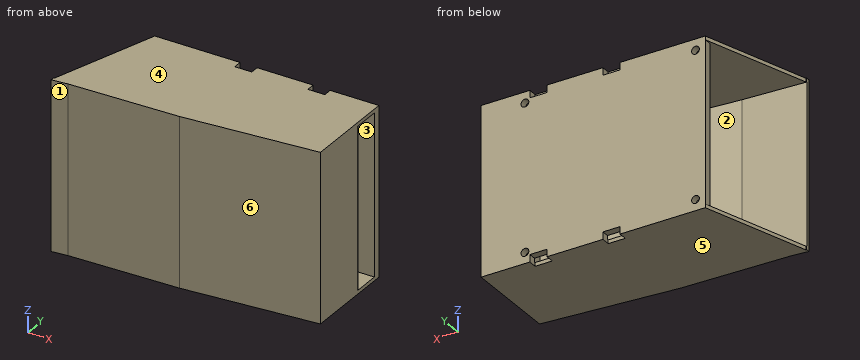
Autodesk Inventor part; units mm, degrees
ref_plane "工作平面1" through (0, 38.6, 0) normal (0, 1, 0) x (-1, 0, 0)
ref_plane "工作平面2" through (0, 0, 34.5) normal (0, 0, -1) x (-1, 0, 0)
ref_plane "工作平面3" through (0, -6, 0) normal (0, 1, 0) x (-1, 0, 0)
sketch "草图1" plane through (0, 0, 0) normal (0, 0, 1) x (1, 0, 0)
  line L0 (0, 0) -> (0, 3)
  line L1 (0, 0) -> (0, -6) construction
  line L2 (0, -6) -> (-106.5, -6) construction
  line L3 (-106.5, -6) -> (0, 3)
  line L4 (0, 0) -> (-54.9206, -4.6412)
  line L5 (-54.9206, -4.6412) -> (-106.5, -6)
  dimension "d0" = 3
  dimension "d1" = 6
  dimension "d2" = 106.5
extrude "拉伸1" add sketch "草图1" along normal blind 69
ref_plane "工作平面1" through (0, 38.6, 0) normal (0, 1, 0) x (-1, 0, 0)
sketch "草图2" plane through (0, 38.6, 0) normal (0, 1, 0) x (-1, 0, 0)
  line L0 (0, 0) -> (106.5, 0) construction
  line L1 (106.5, 0) -> (106.5, 69) construction
  line L2 (0, 69) -> (106.5, 69) construction
  line L3 (0, 0) -> (0, 69) construction
  line L4 (0, 0) -> (92, 0)
  line L5 (92, 0) -> (92, 1.5)
  line L6 (92, 1.5) -> (2, 1.5)
  line L7 (2, 1.5) -> (2, 67.5)
  line L8 (2, 67.5) -> (92, 67.5)
  line L9 (92, 67.5) -> (92, 69)
  line L10 (0, 0) -> (0, 69)
  line L11 (0, 69) -> (92, 69)
  line L12 (0, 69) -> (106.5, 69)
  line L13 (0, 0) -> (0, 69)
  dimension "d6" = 1.5
  dimension "d7" = 1.5
  dimension "d8" = 66
  dimension "d9" = 2
  dimension "d10" = 90
extrude "拉伸2" add sketch "草图2" against normal up to surface from surface at 0 surface through (0, 3, 0) normal (-0.0842069, 0.9964483, 0)
sketch "草图3" plane through (0, 38.6, 0) normal (0, 1, 0) x (-1, 0, 0)
  line L0 (2, 1.5) -> (92, 1.5) construction
  line L1 (2, 67.5) -> (2, 1.5) construction
  line L2 (92, 67.5) -> (2, 67.5) construction
  line L3 (92, 1.5) -> (2, 1.5)
  line L4 (2, 1.5) -> (2, 67.5)
  line L5 (92, 67.5) -> (2, 67.5)
  line L6 (92, 67.5) -> (92, 1.5)
  point P0 (0, 0)
extrude "拉伸3" add sketch "草图3" against normal blind 3
sketch "草图4" plane through (-2, 2.831, 1.5) normal (-1, 0, 0) x (0, 0, 1)
  line L0 (66, 32.769) -> (0, 32.769) construction
  line L1 (0, 0) -> (0, 32.769) construction
  line L2 (66, 0) -> (0, 0) construction
  line L3 (66, 0) -> (66, 32.769) construction
  line L4 (66, -7.6056) -> (66, 32.769)
  line L5 (0, 32.769) -> (66, 32.769)
  line L6 (66, 32.769) -> (66, 22.769)
  line L7 (66, 22.769) -> (0, 22.769)
  line L8 (0, 22.769) -> (0, 32.769)
  point P0 (-1.5, -2.831)
  dimension "d15" = 10
extrude "拉伸4" cut sketch "草图4" against normal through all
sketch "草图5" plane through (0, 0, 69) normal (0, 0, 1) x (1, 0, 0)
  line L0 (-92, -4.7746) -> (-92, 38.6) construction
  line L1 (-92, -4.7746) -> (-106.5, -6) construction
  line L2 (-92, 38.6) -> (-92, -4.7746)
  line L3 (-106.5, -6) -> (-54.9206, -4.6412)
  line L4 (-92, -4.7746) -> (-92, 35.6)
  line L5 (-106.5, -6) -> (-92, -4.7746)
  line L6 (-92, -4.7746) -> (-92, 38.6)
  line L7 (-106.5, -6) -> (-92, 38.6)
  point P0 (0, 0)
extrude "拉伸5" add sketch "草图5" against normal blind 1.5
ref_plane "工作平面2" through (0, 0, 34.5) normal (0, 0, -1) x (-1, 0, 0)
mirror "镜像1" about plane through (0, 0, 34.5) normal (0, 0, -1) of "拉伸5"
sketch "草图7" plane through (0, 38.6, 69) normal (0, 1, 0) x (1, 0, 0)
  line L0 (-92, 69) -> (0, 69)
  line L1 (0, 69) -> (0, 0) construction
  line L2 (0, 34.5) -> (-92.7255, 34.5) construction
  line L3 (-92, 1.5) -> (-92, 67.5)
  point P0 (-18, 64.5)
  point P1 (-52, 64.5)
  point P2 (-88, 64.5)
  point P3 (-18, 4.5)
  point P4 (-52, 4.5)
  point P5 (-88, 4.5)
  point P6 (-92, 66.5)
  dimension "d22" = 4.5
  dimension "d23" = 4.5
  dimension "d24" = 4.5
  dimension "d25" = 34
  dimension "d26" = 36
  dimension "d27" = 60
  dimension "d35" = 4
hole "孔1" at (-88, 38.6, 64.5) at (-88, 38.6, 4.5) at (-18, 38.6, 4.5) at (-18, 38.6, 64.5) direction (0, -1, 0) diameter 3.2 depth 3
fillet "圆角1" radius 1 1 edges at (0, 25.6, 34.5)
sketch "草图9" plane through (0, 0, 69) normal (0, 0, 1) x (1, 0, 0)
  point P0 (0, 0)
sketch "草图10" plane through (0, 0, 69) normal (0, 0, 1) x (1, 0, 0)
  line L0 (-92, 38.6) -> (-106.5, -6) construction
  line L1 (-92, 35.6) -> (-92, 38.6) construction
  line L2 (-92, -4.7746) -> (-92, 35.6) construction
  line L3 (-92, -4.7746) -> (-106.5, -6) construction
  line L4 (-106.5, -6) -> (-54.9206, -4.6412)
  line L5 (-106.5, -6) -> (-106.5, -5)
  line L6 (-127.8168, 0) -> (21.4009, 0)
  line L7 (-106.5, -5) -> (-80.7103, -3.8206)
  line L8 (-2, 2.831) -> (-106.5, -6)
  line L9 (-106.5, -6) -> (-92, 38.6)
  line L10 (-106.5, -6) -> (-80.7103, -3.8206)
  line L11 (-106.5, -6) -> (-106.5, -6.5)
  line L12 (-106.5, -6.5) -> (-80.7103, -3.8206)
  line L13 (-106.5, -5.2) -> (-80.7103, -3.8206)
  point P0 (0, 0)
  dimension "d37" = 1
  dimension "d38" = 25.7897
  dimension "d42" = 0.5
  dimension "d55" = 0.2
extrude "拉伸7" add sketch "草图10" against normal up to surface (69 mm away) from surface at 0 contours L8 L12 L4 | L9 L13 L8 | L5 L13 L9 | L4 L12 L11 | L5 L7 L9 L13 | L13 L9 L7
sketch "草图11" plane through (-54.9206, -4.6412, 0) normal (0.0263351, -0.9996532, 0) x (0.9996532, 0.0263351, 0)
  point P0 (55.0238, 0)
ref_plane "工作平面3" through (0, -6, 0) normal (0, 1, 0) x (-1, 0, 0)
sketch "草图12" plane through (0, 38.6, 69) normal (0, 1, 0) x (1, 0, 0)
  line L0 (0, 0) -> (-92, 0)
  line L1 (-53.5, 0) -> (-53.5, 3)
  line L2 (-92, 1.5) -> (-92, 67.5)
  line L3 (-54.9206, 0) -> (0, 0)
  line L4 (-57, 3) -> (-50, 3)
  line L5 (-50, 3) -> (-50, 0)
  line L6 (-50, 0) -> (-57, 0)
  line L7 (-57, 0) -> (-57, 3)
  line L8 (-92, 1.5) -> (0, 1.5)
  line L9 (-57, 3) -> (-50, 0) construction
  line L10 (-50, 3) -> (-57, 0) construction
  line L11 (-20, 3) -> (-27, 3)
  line L12 (-27, 3) -> (-27, 0)
  line L13 (-27, 0) -> (-20, 0)
  line L14 (-20, 0) -> (-20, 3)
  line L15 (-20, 3) -> (-27, 0) construction
  line L16 (-27, 3) -> (-20, 0) construction
  point P0 (0, 69)
  point P1 (-53.5, 1.5)
  point P2 (-23.5, 1.5)
  dimension "d43" = 38.5
  dimension "d44" = 3
  dimension "d45" = 7
  dimension "d46" = 68.5
  dimension "d47" = 3
  dimension "d48" = 7
extrude "拉伸8" cut sketch "草图12" against normal blind 3.5 contours L0 L12 L8 L14 | L8 L12 L11 L14 | L0 L1 L8 L5 | L0 L7 L8 L1 | L8 L1 L4 L5 | L8 L7 L4 L1
ref_plane "工作平面4" through (0, 0, 34.5) normal (0, 0, 1) x (1, 0, 0)
mirror "镜像2" about plane through (0, 0, 34.5) normal (0, 0, 1) of "拉伸8"
extrude "拉伸9" cut sketch "草图10" along normal up to surface (66 mm away) from surface at -67.5 contours L5 L7 L9 L13 | L13 L9 L7
properties part number "仓库"
CAD build for the part. Positions are in the model's coordinates, mm. Face numbers are marked on the shaded views. A direction names the side the tool comes from. Coordinates: 2 decimals unless noted, no trailing zeros. Write each loop counter-clockwise with the first axis right and the second up, starting at its lowest first coordinate (ties: lowest second). Pieces come first, ordered by that corner, then holes. Notation, with made-up numbers: (19.25, 86.25) -> (53.25, 86.25) arc R22 ccw to (53.25, 94.25) -> close; hole circle Ø4 at (89.25, 69.5). An arc over 180 degrees is marked (long way). Use CSV: the item, a comma, the result in double quotes. Start each with the question number.
Item 1: Band-saw the part on C-C, the plane x = -61.5. Write the cut outline in (y, z), plus the area to 3 significant figures.
Item 2: Wall check: probe 1 along X at (y, z) = (37.45, 64.5); probe 2 along Z at (x, y) = (-18, 36.55); probe 3 along Z at (x, y) = (-50, 0). Give the ranges that are in metal, low to high.
Item 3: Drop flat-ended pins along their axis: P1, Ø3.5, axis at x = -24.5, y = 37.5, coming from the +Z side; P2, Ø2.5, axis at x = -88, z = 64.5, coming from the +Y side; P3, Ø3, axis at x = -18, z = 4.5, coming from the -Y side; P4, Ø4, axis at y = 28, z = 32, coming from the -X side. Give the stop position or say it passes through.
Item 4: Tool access for the marked faces 1 and 2: list every direction of +Z, -Z, +X, -X, +Y, -Y with a clear straight run to the whole face (end or side of a thin tool).
Item 5: Band-saw the part on B-B, the plane z = 28. Write the cut outline in (x, y).
Item 6: Band-saw the part on A-A, the plane z = 4.5. Write the cut outline in (x, y).
Item 7: Band-saw the part on D-D, the plane y = 23.5. Write the cut outline in (x, z).
Item 8: Two-plate mould, pull along Z, no slides. Class the marked faces 3, 4, 5 and 6: +Z half, -Z half, draft (parallel to the pull), parting line (faces both ways), or undercut.
Response values:
1,outline,"(-4.81, 0) -> (38.6, 0) -> (38.6, 69) -> (-4.81, 69) -> close; hole (-2.2, 1.5) -> (35.6, 1.5) -> (35.6, 67.5) -> (-2.2, 67.5) -> close"
1,area,"501 mm2"
2,probe 1,"x = -92 to -89.6, -86.4 to -19.6, -16.4 to 0"
2,probe 2,"z = 0 to 2.9, 6.1 to 62.9, 66.1 to 69"
2,probe 3,"z = 0 to 1.5, 67.5 to 69"
3,P1,"stops at z = 66"
3,P2,"stops at y = -4.14"
3,P3,"stops at y = -1.65"
3,P4,"passes through"
4,face 1,"+Z, -Z, +X, -Y"
4,face 2,"-X"
5,outline,"(-106.5, -6.5) -> (-100.05, -5.83) -> (-54.92, -4.64) -> (0, 0) -> (0, 24.6) arc R1 ccw to (-1, 25.6) -> (-2, 25.6) -> (-2, 2.83) -> (-80.71, -3.82) -> (-106.5, -5.2) -> close; (-92, 35.6) -> (0, 35.6) -> (0, 38.6) -> (-92, 38.6) -> close"
6,outline,"(-106.5, -6.5) -> (-100.05, -5.83) -> (-54.92, -4.64) -> (0, 0) -> (0, 24.6) arc R1 ccw to (-1, 25.6) -> (-2, 25.6) -> (-2, 2.83) -> (-80.71, -3.82) -> (-106.5, -5.2) -> close; (-92, 35.6) -> (-89.6, 35.6) -> (-89.6, 38.6) -> (-92, 38.6) -> close; (-86.4, 35.6) -> (-19.6, 35.6) -> (-19.6, 38.6) -> (-86.4, 38.6) -> close; (-16.4, 35.6) -> (0, 35.6) -> (0, 38.6) -> (-16.4, 38.6) -> close"
7,outline,"(-96.91, 0) -> (0, 0) -> (0, 69) -> (-96.91, 69) -> (-96.91, 67.5) -> (-2, 67.5) -> (-2, 1.5) -> (-96.91, 1.5) -> close"
8,face 3,"undercut"
8,face 4,"+Z half"
8,face 5,"-Z half"
8,face 6,"draft"
